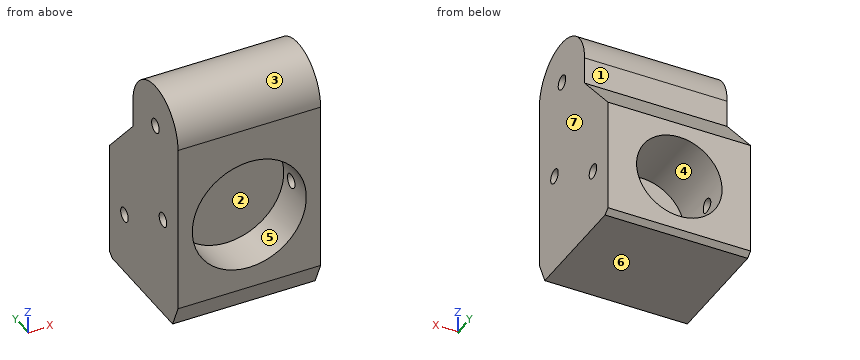
```python
from build123d import *

# Parameters (mm, degrees)
SKETCH1_W           = 120
SKETCH1_H           = 60
BOSS_EXTRUDE1_DEPTH = 100
SKETCH2_R           = 40
CUT_EXTRUDE1_DEPTH  = 30
SKETCH3_R           = 5
CUT_EXTRUDE2_DEPTH  = 121.415945788
BOSS_EXTRUDE2_DEPTH = 100
SKETCH9_R           = 30
CUT_EXTRUDE6_DEPTH  = 50
SKETCH5_R           = 5
CUT_EXTRUDE3_DEPTH  = 100


with BuildPart() as part:
    # Sketch1 → Boss-Extrude1 (new body)
    with BuildSketch(Plane(origin=(0, 0, 0), x_dir=(0, 0, -1), z_dir=(1, 0, 0))):
        Rectangle(SKETCH1_W, SKETCH1_H)
    extrude(amount=-BOSS_EXTRUDE1_DEPTH)

    # Sketch2 → Cut-Extrude1 (cut)
    with BuildSketch(Plane.XZ.offset(30)):
        with Locations(Location((-50, -5, 0), (0, 0, 270))):
            Circle(SKETCH2_R)
    extrude(amount=-CUT_EXTRUDE1_DEPTH, mode=Mode.SUBTRACT)

    # Sketch3 → Cut-Extrude2 (cut, through all)
    with BuildSketch(Plane(origin=(0, 0, 0), x_dir=(0, 0, -1), z_dir=(1, 0, 0))):
        with Locations((5, -10)):
            Circle(SKETCH3_R)
    extrude(amount=-CUT_EXTRUDE2_DEPTH, mode=Mode.SUBTRACT)

    # Sketch4 → Boss-Extrude2 (add)
    with BuildSketch(Plane(origin=(0, 0, 0), x_dir=(0, 0, -1), z_dir=(1, 0, 0))):
        with BuildLine():
            Line((-60, 30), (-60, -30))
            ThreePointArc((-60, -30), (-90, 0), (-60, 30))
        make_face()
        Polygon((60, 30), (60, -30), (76, -22.836697104), (76, 57.163302896), (72.921242275, 61.103004772), (-7.078757725, 61.103004772), (-40.915642919, 30), align=None)
    extrude(amount=-BOSS_EXTRUDE2_DEPTH)

    # Sketch9 → Cut-Extrude6 (cut)
    with BuildSketch(Plane(origin=(0, 61.103004772, 0), x_dir=(1, 0, 0), z_dir=(0, 1, 0))):
        with Locations(Location((-50, 32.921242275, 0), (0, 0, 270))):
            Circle(SKETCH9_R)
    extrude(amount=-CUT_EXTRUDE6_DEPTH, mode=Mode.SUBTRACT)

    # Sketch5 → Cut-Extrude3 (cut)
    with BuildSketch(Plane(origin=(0, 0, 0), x_dir=(0, 0, -1), z_dir=(1, 0, 0))):
        with Locations((-60, 0)):
            Circle(SKETCH5_R)
        with Locations((32.921242275, 41.103004772)):
            Circle(SKETCH5_R)
    extrude(amount=-CUT_EXTRUDE3_DEPTH, mode=Mode.SUBTRACT)


solid = part.part
```
The listing builds one solid part. Answer for the finished solid, in the listing's coordinates (mm). Face numbers are marked on the shaded views. A direction names the side the tool comes from. Coordinates: 2 decimals unless noted, no trailing zeros. Order: outer loops, then holes, each group sorted by start corner. A loop starts at its lowest first (then second) coordinate and runs counter-clockwise, first axis right, second up. Notation, with made-up numbers: M 70,75.25 L 98,75.25 A32 ccw 98,109.25 Z; hole C 5.5,33 d9. An arc over 180 degrees is marked long. Answer as a JSON object with one key per item and string values. Group by question number.
1. Section C-C on x = -94 is taken. Write down the section's boundary in (y, z), then the cut area to 3 significant figures.
2. Section A-A on x = -50 is taken. Write down the section's boundary in (y, z).
3. Flat-ended cylindrical pins translate along their axes: P1, Ø4, axis at x = -82.5, y = 12, coming from the +Z side; P2, Ø12, axis at x = -47, z = -26.5, coming from the +Y side; P3, Ø1, axis at x = -90, y = 34.5, coming from the +Z side. Find the tip coordinate at first contact, or state that the pin passes through.
4. A tool of negligible diameter and unlimited length cuts with its end or side. For the marked faces 1, 2, 3 and 4, from which of +Z, -Z, +X, -X, +Y, -Y can it reach the whole face along a straight path? Write none if from no direction.
5. Straight lines are drawn through the part: line 1 (Y direction, x = -94, z = -5); line 2 (X direction, y = -21.5, z = -5); line 3 (Y direction, x = -51, z = 60). For each, find the intervals that lie inside material, in ascending order.
6. Determine the mould class of the marked faces 5, 6 and 7 for opening direction Z: released by +Z, released by -Z, zero draft, split by the parting line, or undercut.
7. Section B-B on y = -10 is taken. Write down the section's boundary in (x, z).
8. Section D-D on y = 26 is taken. Write down the section's boundary in (x, z).
Values follow:
{
 "1": {"outline": "M -30,-60 L -22.84,-76 L 57.16,-76 L 61.1,-72.92 L 61.1,7.08 L 30,40.92 L 30,60 A30 ccw -30,60 Z; hole C -10,-5 d10; hole C 0,60 d10; hole C 41.1,-32.92 d10", "area": "12,400 mm2"},
 "2": {"outline": "M -30,-60 L -22.84,-76 L 57.16,-76 L 61.1,-72.92 L 61.1,-62.92 L 11.1,-62.92 L 11.1,-2.92 L 61.1,-2.92 L 61.1,7.08 L 30,40.92 L 30,60 A30 ccw -30,60 L -30,35 L 0,35 L 0,-45 L -30,-45 Z; hole C 0,60 d10"},
 "3": {"P1": "z = 88.28", "P2": "y = 11.1", "P3": "z = 36.56"},
 "4": {"face 1": "+Z, +X, -X, +Y", "face 2": "-Y", "face 3": "+Z, +X, -X", "face 4": "+Y"},
 "5": {"line 1": "-30 to -15, -5 to 61.1", "line 2": "-100 to -90, -10 to 0", "line 3": "-30 to -5, 5 to 30"},
 "6": {"face 5": "undercut", "face 6": "released by -Z", "face 7": "zero draft"},
 "7": {"outline": "M -100,-76 L 0,-76 L 0,-10 L -10.31,-10 A40 cw -89.69,-10 L -100,-10 Z; M -100,0 L -89.69,0 A40 cw -10.31,0 L 0,0 L 0,88.28 L -100,88.28 Z"},
 "8": {"outline": "M -100,-76 L 0,-76 L 0,74.97 L -100,74.97 Z; hole C -50,-32.92 d60"}
}
